from build123d import *

# Parameters (mm, degrees)
F0_R     = 1.6
F1_DEPTH = 4


with BuildPart() as f1:
    # F0 (on Top) → F1 (new body)
    with BuildSketch(Plane.XY):
        with BuildLine():
            Line((-44.408627, -61.525488), (-44.408627, -91.060406))
            Line((-44.408627, -91.060406), (-40.651218, -91.32315))
            ThreePointArc((-40.651218, -91.32315), (-37.343231, -92.900978), (-36, -96.31097))
            Line((-36, -96.31097), (-36, -96.648395))
            ThreePointArc((-36, -96.648395), (-34.535534, -100.183929), (-31, -101.648395))
            Line((-31, -101.648395), (0, -101.648395))
            Line((0, -101.648395), (31, -101.648395))
            ThreePointArc((31, -101.648395), (34.535534, -100.183929), (36, -96.648395))
            Line((36, -96.648395), (36, -96.31097))
            ThreePointArc((36, -96.31097), (37.343231, -92.900978), (40.651218, -91.32315))
            Line((40.651218, -91.32315), (44.408627, -91.060406))
            Line((44.408627, -91.060406), (44.408627, -61.525488))
            Line((44.408627, -61.525488), (39.450638, -61.178791))
            ThreePointArc((39.450638, -61.178791), (36.142652, -59.600963), (34.799421, -56.190971))
            Line((34.799421, -56.190971), (34.799421, 0))
            Line((34.799421, 0), (34.799421, 56.190971))
            ThreePointArc((34.799421, 56.190971), (36.142652, 59.600963), (39.450638, 61.178791))
            Line((39.450638, 61.178791), (44.408627, 61.525488))
            Line((44.408627, 61.525488), (44.408627, 91.060406))
            Line((44.408627, 91.060406), (40.651218, 91.32315))
            ThreePointArc((40.651218, 91.32315), (37.343231, 92.900978), (36, 96.31097))
            Line((36, 96.31097), (36, 96.648395))
            ThreePointArc((36, 96.648395), (34.535534, 100.183929), (31, 101.648395))
            Line((31, 101.648395), (0, 101.648395))
            Line((0, 101.648395), (-31, 101.648395))
            ThreePointArc((-31, 101.648395), (-34.535534, 100.183929), (-36, 96.648395))
            Line((-36, 96.648395), (-36, 96.31097))
            ThreePointArc((-36, 96.31097), (-37.343231, 92.900978), (-40.651218, 91.32315))
            Line((-40.651218, 91.32315), (-44.408627, 91.060406))
            Line((-44.408627, 91.060406), (-44.408627, 61.525488))
            Line((-44.408627, 61.525488), (-39.450638, 61.178791))
            ThreePointArc((-39.450638, 61.178791), (-36.142652, 59.600963), (-34.799421, 56.190971))
            Line((-34.799421, 56.190971), (-34.799421, 0))
            Line((-34.799421, 0), (-34.799421, -56.190971))
            ThreePointArc((-34.799421, -56.190971), (-36.142652, -59.600963), (-39.450638, -61.178791))
            Line((-39.450638, -61.178791), (-44.408627, -61.525488))
        make_face()
        with Locations((-39.408627, -84.392947)):
            Circle(F0_R, mode=Mode.SUBTRACT)
        with Locations((-23.110468, -76.292947)):
            Circle(F0_R, mode=Mode.SUBTRACT)
        with Locations((-39.408627, -68.192947)):
            Circle(F0_R, mode=Mode.SUBTRACT)
        with BuildLine():
            ThreePointArc((-22.877386, -42.681136), (-23.609619, -44.448903), (-25.377386, -45.181136))
            ThreePointArc((-25.377386, -45.181136), (-27.145153, -44.448903), (-27.877386, -42.681136))
            Line((-27.877386, -42.681136), (-27.877386, -12.681136))
            ThreePointArc((-27.877386, -12.681136), (-27.145153, -10.913369), (-25.377386, -10.181136))
            ThreePointArc((-25.377386, -10.181136), (-23.609619, -10.913369), (-22.877386, -12.681136))
            Line((-22.877386, -12.681136), (-22.877386, -42.681136))
        make_face(mode=Mode.SUBTRACT)
        with BuildLine():
            ThreePointArc((-9.422034, -10.181136), (-7.654267, -10.913369), (-6.922034, -12.681136))
            Line((-6.922034, -12.681136), (-6.922034, -42.681136))
            ThreePointArc((-6.922034, -42.681136), (-7.654267, -44.448903), (-9.422034, -45.181136))
            ThreePointArc((-9.422034, -45.181136), (-11.189801, -44.448903), (-11.922034, -42.681136))
            Line((-11.922034, -42.681136), (-11.922034, -12.681136))
            ThreePointArc((-11.922034, -12.681136), (-11.189801, -10.913369), (-9.422034, -10.181136))
        make_face(mode=Mode.SUBTRACT)
        Polygon((16.318487, -65.480797), (16.364526, -84.350343), (0.046039, -93.824987), (-16.318487, -84.430085), (-16.364526, -65.560539), (-0.046039, -56.085895), align=None, mode=Mode.SUBTRACT)
        with Locations((23.110468, -76.292947)):
            Circle(F0_R, mode=Mode.SUBTRACT)
        with Locations((39.408627, -84.392947)):
            Circle(F0_R, mode=Mode.SUBTRACT)
        with Locations((39.408627, -68.192947)):
            Circle(F0_R, mode=Mode.SUBTRACT)
        with BuildLine():
            ThreePointArc((6.922034, -12.681136), (7.654267, -10.913369), (9.422034, -10.181136))
            ThreePointArc((9.422034, -10.181136), (11.189801, -10.913369), (11.922034, -12.681136))
            Line((11.922034, -12.681136), (11.922034, -42.681136))
            ThreePointArc((11.922034, -42.681136), (11.189801, -44.448903), (9.422034, -45.181136))
            ThreePointArc((9.422034, -45.181136), (7.654267, -44.448903), (6.922034, -42.681136))
            Line((6.922034, -42.681136), (6.922034, -12.681136))
        make_face(mode=Mode.SUBTRACT)
        with BuildLine():
            ThreePointArc((25.377386, -45.181136), (23.609619, -44.448903), (22.877386, -42.681136))
            Line((22.877386, -42.681136), (22.877386, -12.681136))
            ThreePointArc((22.877386, -12.681136), (23.609619, -10.913369), (25.377386, -10.181136))
            ThreePointArc((25.377386, -10.181136), (27.145153, -10.913369), (27.877386, -12.681136))
            Line((27.877386, -12.681136), (27.877386, -42.681136))
            ThreePointArc((27.877386, -42.681136), (27.145153, -44.448903), (25.377386, -45.181136))
        make_face(mode=Mode.SUBTRACT)
        with BuildLine():
            ThreePointArc((-22.877386, 12.681136), (-23.609619, 10.913369), (-25.377386, 10.181136))
            ThreePointArc((-25.377386, 10.181136), (-27.145153, 10.913369), (-27.877386, 12.681136))
            Line((-27.877386, 12.681136), (-27.877386, 42.681136))
            ThreePointArc((-27.877386, 42.681136), (-27.145153, 44.448903), (-25.377386, 45.181136))
            ThreePointArc((-25.377386, 45.181136), (-23.609619, 44.448903), (-22.877386, 42.681136))
            Line((-22.877386, 42.681136), (-22.877386, 12.681136))
        make_face(mode=Mode.SUBTRACT)
        with BuildLine():
            Line((-6.922034, 42.681136), (-6.922034, 12.681136))
            ThreePointArc((-6.922034, 12.681136), (-7.654267, 10.913369), (-9.422034, 10.181136))
            ThreePointArc((-9.422034, 10.181136), (-11.189801, 10.913369), (-11.922034, 12.681136))
            Line((-11.922034, 12.681136), (-11.922034, 42.681136))
            ThreePointArc((-11.922034, 42.681136), (-11.189801, 44.448903), (-9.422034, 45.181136))
            ThreePointArc((-9.422034, 45.181136), (-7.654267, 44.448903), (-6.922034, 42.681136))
        make_face(mode=Mode.SUBTRACT)
        with Locations((-39.408627, 68.192947)):
            Circle(F0_R, mode=Mode.SUBTRACT)
        with Locations((-39.408627, 84.392947)):
            Circle(F0_R, mode=Mode.SUBTRACT)
        with Locations((-23.110468, 76.292947)):
            Circle(F0_R, mode=Mode.SUBTRACT)
        with BuildLine():
            ThreePointArc((9.422034, 10.181136), (7.654267, 10.913369), (6.922034, 12.681136))
            Line((6.922034, 12.681136), (6.922034, 42.681136))
            ThreePointArc((6.922034, 42.681136), (7.654267, 44.448903), (9.422034, 45.181136))
            ThreePointArc((9.422034, 45.181136), (11.189801, 44.448903), (11.922034, 42.681136))
            Line((11.922034, 42.681136), (11.922034, 12.681136))
            ThreePointArc((11.922034, 12.681136), (11.189801, 10.913369), (9.422034, 10.181136))
        make_face(mode=Mode.SUBTRACT)
        with BuildLine():
            ThreePointArc((22.877386, 42.681136), (23.609619, 44.448903), (25.377386, 45.181136))
            ThreePointArc((25.377386, 45.181136), (27.145153, 44.448903), (27.877386, 42.681136))
            Line((27.877386, 42.681136), (27.877386, 12.681136))
            ThreePointArc((27.877386, 12.681136), (27.145153, 10.913369), (25.377386, 10.181136))
            ThreePointArc((25.377386, 10.181136), (23.609619, 10.913369), (22.877386, 12.681136))
            Line((22.877386, 12.681136), (22.877386, 42.681136))
        make_face(mode=Mode.SUBTRACT)
        Polygon((-0.046039, 56.085895), (-16.364526, 65.560539), (-16.318487, 84.430085), (0.046039, 93.824987), (16.364526, 84.350343), (16.318487, 65.480797), align=None, mode=Mode.SUBTRACT)
        with Locations((39.408627, 68.192947)):
            Circle(F0_R, mode=Mode.SUBTRACT)
        with Locations((23.110468, 76.292947)):
            Circle(F0_R, mode=Mode.SUBTRACT)
        with Locations((39.408627, 84.392947)):
            Circle(F0_R, mode=Mode.SUBTRACT)
    extrude(amount=F1_DEPTH)


solid = f1.part
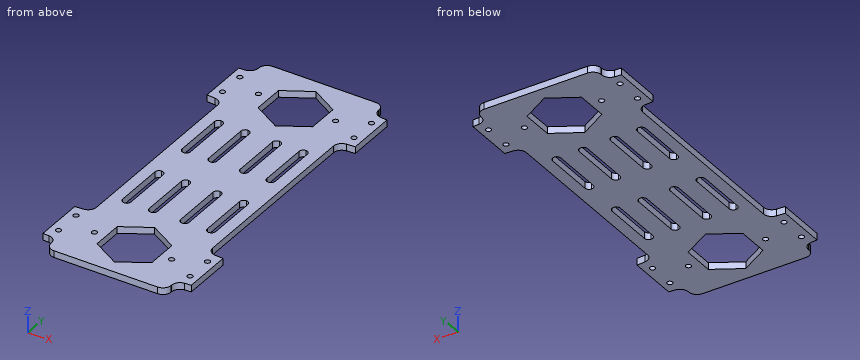
Check sheet for the modelled part. Datum: model origin and axes. Units: mm. Round coordinates to 2 decimals unless told otherwise and drop trailing zeros. Write each loop counter-clockwise with the first axis right and the second up, starting at its lowest first coordinate (ties: lowest second). Pieces come first, ordered by that corner, then holes. Notation, with made-up numbers: (-37, 11) - (17, 11) arc R11 ccw to (17, 23) - close; hole circle Ø7 at (67, -24.75). An arc over 180 degrees is marked (long way). Return JSON: item names as keys, results as strings.
Q1. Cross-section at B-B (y = -22). Record the boundary of the cut face in (x, z).
Returned:
{"outline": "(-34.8, 0) - (-27.88, 0) - (-27.88, 4) - (-34.8, 4) - close; (-22.88, 0) - (-11.92, 0) - (-11.92, 4) - (-22.88, 4) - close; (-6.92, 0) - (6.92, 0) - (6.92, 4) - (-6.92, 4) - close; (11.92, 0) - (22.88, 0) - (22.88, 4) - (11.92, 4) - close; (27.88, 0) - (34.8, 0) - (34.8, 4) - (27.88, 4) - close"}
Q2. Cross-section at C-C (z = 0.7). Give the number of separate pieces and of enclosed holes in the cut face, then the cut area to 3 significant figures.
Returned:
{"separate pieces": "1", "enclosed holes": "22", "area": "12,100 mm²"}
Q3. Scan lines: L1, parallel to X at y = 31.5, z = 0.9; L2, parallel to Y at x = -3, z = 2.65; L3, parallel to Y at x = -27, z = 2.8. Record each from-to range of solid material in increasing order. Write a range as from..to.
Returned:
{"L1": "x = -34.8..-27.88, -22.88..-11.92, -6.92..6.92, 11.92..22.88, 27.88..34.8", "L2": "y = -101.65..-92.08, -57.8..57.8, 92.08..101.65", "L3": "y = -101.65..-44.58, -10.78..10.78, 44.58..101.65"}
Q4. Cross-section at A-A (y = 59). Record the boundary of the cut face in (x, z).
Returned:
{"outline": "(-35.66, 0) - (-5.07, 0) - (-5.07, 4) - (-35.66, 4) - close; (5.03, 0) - (35.66, 0) - (35.66, 4) - (5.03, 4) - close"}
Q5. Depth check by flat-ended pin: P1, Ø2, axis at y = 33, z = 1.5, coming from the -X side; P2, Ø1, axis at x = -32, z = 2.5, coming from the +Y side; P3, Ø1.2, axis at y = -20.5, z = 3, coming from the +X side. Enter the tip coordinate at first touch or a pass-through.
Returned:
{"P1": "stops at x = -34.8", "P2": "stops at y = 101.62", "P3": "stops at x = 34.8"}
